Source: CAD feature listing. Evaluate the final solid. Frame: model axes, mm. Coordinates: 2 decimals unless noted, no trailing zeros. Write each loop counter-clockwise with the first axis right and the second up, starting at its lowest first coordinate (ties: lowest second). Pieces come first, ordered by that corner, then holes. Notation, with made-up numbers: M -28.75,32 L 26.25,32 A21 ccw 26.25,50 Z; hole C 84,5 d7. An arc over 180 degrees is marked long. One line per item, written item: value. Start each with the question number.
Item 1: Ray query, L1, parallel to Y at x = 125.5, z = 1.55. Return the intervals inside material, ascending. Write a range as from..to.
Item 2: Cut plane B-B, the plane y = 283. State how many separate pieces and enclosed holes the cut face has, then the cut area to 3 significant figures.
Item 3: Cut plane A-A, the plane x = 65. Output: boundary loops of the cut face in (y, z), then the cut area to 3 significant figures.
```python
from build123d import *

# Parameters (mm, degrees)
MODEL_W             = 147
MODEL_H             = 71
MODEL_W_2           = 14
MODEL_H_2           = 14
BOSS_EXTRUDE1_DEPTH = 2
BREAK_CORNER1_DEPTH = 2


# Read off the part's stored shape, not the designer's step: Break-Corner1
with BuildPart() as part:
    # Model → Boss-Extrude1 (new body)
    with BuildSketch(Plane.XY):
        with Locations((125.770541641, 281.208862918)):
            Rectangle(MODEL_W, MODEL_H)
        with Locations((125.770541641, 262.208862918)):
            Rectangle(MODEL_W_2, MODEL_H_2, mode=Mode.SUBTRACT)
        with Locations((125.770541641, 281.208862918)):
            Rectangle(MODEL_W_2, MODEL_H_2, mode=Mode.SUBTRACT)
        with Locations((125.770541641, 300.208862918)):
            Rectangle(MODEL_W_2, MODEL_H_2, mode=Mode.SUBTRACT)
        with Locations((107.146916797, 300.208862918)):
            Rectangle(MODEL_W_2, MODEL_H_2, mode=Mode.SUBTRACT)
        with Locations((88.146916797, 300.208862918)):
            Rectangle(MODEL_W_2, MODEL_H_2, mode=Mode.SUBTRACT)
        with Locations((69.146916797, 300.208862918)):
            Rectangle(MODEL_W_2, MODEL_H_2, mode=Mode.SUBTRACT)
        with Locations((69.146916797, 281.208862918)):
            Rectangle(MODEL_W_2, MODEL_H_2, mode=Mode.SUBTRACT)
        with Locations((69.146916797, 262.208862918)):
            Rectangle(MODEL_W_2, MODEL_H_2, mode=Mode.SUBTRACT)
        with Locations((88.146916797, 281.208862918)):
            Rectangle(MODEL_W_2, MODEL_H_2, mode=Mode.SUBTRACT)
        with Locations((107.146916797, 281.208862918)):
            Rectangle(MODEL_W_2, MODEL_H_2, mode=Mode.SUBTRACT)
        with Locations((88.146916797, 262.208862918)):
            Rectangle(MODEL_W_2, MODEL_H_2, mode=Mode.SUBTRACT)
        with Locations((107.146916797, 262.208862918)):
            Rectangle(MODEL_W_2, MODEL_H_2, mode=Mode.SUBTRACT)
        with Locations((182.770541641, 300.208862918)):
            Rectangle(MODEL_W_2, MODEL_H_2, mode=Mode.SUBTRACT)
        with Locations((163.770541641, 300.208862918)):
            Rectangle(MODEL_W_2, MODEL_H_2, mode=Mode.SUBTRACT)
        with Locations((144.770541641, 300.208862918)):
            Rectangle(MODEL_W_2, MODEL_H_2, mode=Mode.SUBTRACT)
        with Locations((144.770541641, 281.208862918)):
            Rectangle(MODEL_W_2, MODEL_H_2, mode=Mode.SUBTRACT)
        with Locations((144.770541641, 262.208862918)):
            Rectangle(MODEL_W_2, MODEL_H_2, mode=Mode.SUBTRACT)
        with Locations((163.770541641, 281.208862918)):
            Rectangle(MODEL_W_2, MODEL_H_2, mode=Mode.SUBTRACT)
        with Locations((182.770541641, 281.208862918)):
            Rectangle(MODEL_W_2, MODEL_H_2, mode=Mode.SUBTRACT)
        with Locations((163.770541641, 262.208862918)):
            Rectangle(MODEL_W_2, MODEL_H_2, mode=Mode.SUBTRACT)
        with Locations((182.770541641, 262.208862918)):
            Rectangle(MODEL_W_2, MODEL_H_2, mode=Mode.SUBTRACT)
    extrude(amount=BOSS_EXTRUDE1_DEPTH)

    # Break-Corner1 outline → Break-Corner1 (cut)
    with BuildSketch(Plane.XY):
        with BuildLine():
            Line((199.270541641, 245.708862918), (199.270541641, 247.708862918))
            ThreePointArc((199.270541641, 247.708862918), (198.684755203, 246.294649356), (197.270541641, 245.708862918))
            Line((197.270541641, 245.708862918), (199.270541641, 245.708862918))
        make_face()
        with BuildLine():
            ThreePointArc((197.270541641, 316.708862918), (198.684755204, 316.123076481), (199.270541641, 314.708862918))
            Line((199.270541641, 314.708862918), (199.270541641, 316.708862918))
            Line((199.270541641, 316.708862918), (197.270541641, 316.708862918))
        make_face()
        with BuildLine():
            Line((52.270541641, 245.708862918), (54.270541641, 245.708862918))
            ThreePointArc((54.270541641, 245.708862918), (52.856328079, 246.294649356), (52.270541641, 247.708862918))
            Line((52.270541641, 247.708862918), (52.270541641, 245.708862918))
        make_face()
        with BuildLine():
            ThreePointArc((52.270541641, 314.708862918), (52.856328079, 316.123076481), (54.270541641, 316.708862918))
            Line((54.270541641, 316.708862918), (52.270541641, 316.708862918))
            Line((52.270541641, 316.708862918), (52.270541641, 314.708862918))
        make_face()
    extrude(amount=BREAK_CORNER1_DEPTH, mode=Mode.SUBTRACT)


solid = part.part
```
From the geometry:
1. L1: y = 245.71..255.21, 269.21..274.21, 288.21..293.21, 307.21..316.71
2. separate pieces: 8
2. enclosed holes: 0
2. area: 98.0 mm²
3. outline: M 245.71,0 L 255.21,0 L 255.21,2 L 245.71,2 Z; M 269.21,0 L 274.21,0 L 274.21,2 L 269.21,2 Z; M 288.21,0 L 293.21,0 L 293.21,2 L 288.21,2 Z; M 307.21,0 L 316.71,0 L 316.71,2 L 307.21,2 Z
3. area: 58.0 mm²
